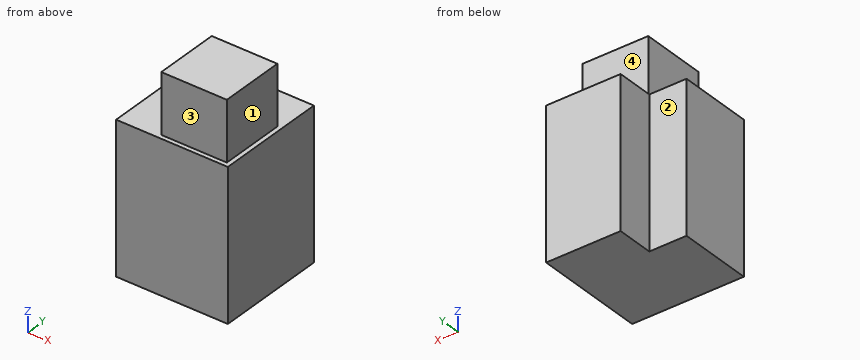
```python
from build123d import *

# Parameters (mm, degrees)
BOX_W              = 10
BOX_H              = 10
BOX_DEPTH          = 10
SKETCH_W           = 4.4
SKETCH_H           = 4.4
PAD_DEPTH          = 4
PAD_FACE4_W        = 10
PAD_FACE4_H        = 10
POCKET_DEPTH       = 2.5
POCKET_FACE5_W     = 10
POCKET_FACE5_H     = 10
POCKET001_DEPTH    = 2.5
SKETCH001_W        = 5
SKETCH001_H        = 10
PAD001_DEPTH       = 10
SKETCH002_W        = 4.4
SKETCH002_H        = 4.4
PAD002_DEPTH       = 4
PAD002_FACE22_W    = 4.4
PAD002_FACE22_H    = 4.4
POCKET002_DEPTH    = 5
POCKET002_FACE16_W = 5
POCKET002_FACE16_H = 10
POCKET003_DEPTH    = 7.5
POCKET003_FACE7_W  = 2.5
POCKET003_FACE7_H  = 10
POCKET004_DEPTH    = 5


with BuildPart() as part:
    # Box → Box (new body)
    with BuildSketch(Plane.XY):
        with Locations((5, 5)):
            Rectangle(BOX_W, BOX_H)
    extrude(amount=BOX_DEPTH)

    # Sketch (on Face6 of BaseFeature) → Pad (new body)
    with BuildSketch(Plane.XY.offset(10)):
        with Locations((5, 5)):
            Rectangle(SKETCH_W, SKETCH_H)
    extrude(amount=PAD_DEPTH)

    # Pad Face4 → Pocket (cut)
    with BuildSketch(Plane(origin=(5, 10, 5), x_dir=(1, 0, 0), z_dir=(0, 1, 0))):
        Rectangle(PAD_FACE4_W, PAD_FACE4_H)
    extrude(amount=-POCKET_DEPTH, mode=Mode.SUBTRACT)

    # Pocket Face5 → Pocket001 (cut)
    with BuildSketch(Plane(origin=(5, 0, 5), x_dir=(-1, 0, 0), z_dir=(0, -1, 0))):
        Rectangle(POCKET_FACE5_W, POCKET_FACE5_H)
    extrude(amount=-POCKET001_DEPTH, mode=Mode.SUBTRACT)

    # Sketch001 (on Face3 of Pocket001) → Pad001 (join)
    with BuildSketch(Plane(origin=(0, 7.5, 0), x_dir=(-1, 0, 0), z_dir=(0, 1, 0))):
        with Locations((-5, 5)):
            Rectangle(SKETCH001_W, SKETCH001_H)
    extrude(amount=PAD001_DEPTH)

    # Sketch002 (on Face6 of Pad001) → Pad002 (join)
    with BuildSketch(Plane.XY.offset(10)):
        with Locations((5, 12.5)):
            Rectangle(SKETCH002_W, SKETCH002_H)
    extrude(amount=PAD002_DEPTH)

    # Pad002 Face22 → Pocket002 (cut)
    with BuildSketch(Plane(origin=(5, 12.5, 14), x_dir=(0, 1, 0), z_dir=(0, 0, 1))):
        Rectangle(PAD002_FACE22_W, PAD002_FACE22_H)
    extrude(amount=-POCKET002_DEPTH, mode=Mode.SUBTRACT)

    # Pocket002 Face16 → Pocket003 (cut)
    with BuildSketch(Plane(origin=(5, 17.5, 5), x_dir=(1, 0, 0), z_dir=(0, 1, 0))):
        Rectangle(POCKET002_FACE16_W, POCKET002_FACE16_H)
    extrude(amount=-POCKET003_DEPTH, mode=Mode.SUBTRACT)

    # Pocket003 Face7 → Pocket004 (cut)
    with BuildSketch(Plane(origin=(8.75, 7.5, 5), x_dir=(1, 0, 0), z_dir=(0, 1, 0))):
        Rectangle(POCKET003_FACE7_W, POCKET003_FACE7_H)
    extrude(amount=-POCKET004_DEPTH, mode=Mode.SUBTRACT)


solid = part.part
```
Work out the finished part from the listing and answer in its coordinate system (mm). Face numbers are marked on the shaded views. A direction names the side the tool comes from. Coordinates: 2 decimals unless noted, no trailing zeros. Loops run counter-clockwise (first coordinate to the right, second up) from the corner with the lowest first, then second, coordinate; pieces in that order, holes last. Notation, with made-up numbers: (35.5, 48.5) -> (58.5, 48.5) arc R17 cw to (58.5, 78.5) -> close; hole circle Ø3 at (59, 8). An arc over 180 degrees is marked (long way). Answer as CSV lines item,"result".
Q1. The part is cut by section A-A on x = 5. Write down the section's boundary in (y, z), and give its area (3 significant figures).
Findings:
outline,"(2.5, 0) -> (10, 0) -> (10, 10) -> (7.2, 10) -> (7.2, 14) -> (2.8, 14) -> (2.8, 10) -> (2.5, 10) -> close"
area,"92.6 mm²"
Q2. The part is cut by section C-C on z = 6.75. Write down the section's boundary in (x, y), and give its area (3 significant figures).
Findings:
outline,"(0, 2.5) -> (7.5, 2.5) -> (7.5, 10) -> (2.5, 10) -> (2.5, 7.5) -> (0, 7.5) -> close"
area,"50.0 mm²"
Q3. A tool of negligible diameter and unlimited length cuts with its end or side. For the marked faces 1, 2, 3 and 4, from which of +Z, -Z, +X, -X, +Y, -Y can it reach the whole face along a straight path? Write none if from no direction.
Findings:
face 1,"+Z, +X, +Y, -Y"
face 2,"+Z, -Z, -X, +Y"
face 3,"+Z, +X, -X, -Y"
face 4,"+Z, +X, -X, +Y"
Q4. Find the intervals of material crossed by probe 1 along Y at (x, z) = (4.75, 11.75); probe 2 along Y at (x, z) = (1.5, 4.5); probe 3 along Z at (x, y) = (3, 7.75), in increasing order.
Findings:
probe 1,"y = 2.8 to 7.2"
probe 2,"y = 2.5 to 7.5"
probe 3,"z = 0 to 10"
Q5. Each of these flat-tipped pins is pushed along its axis until it touches: pin 1 (3 mm diameter, centred on x = 4.5, y = 5.5, fed in from -Z); pin 2 (1.2 mm diameter, centred on x = 1, z = 6, fed in from +Y); pin 3 (3 mm diameter, centred on y = 4, z = 12, fed in from -X); pin 4 (2 mm diameter, centred on x = 4.5, z = 13, fed in from -Y). Where does it stop, or does it pass through?
Findings:
pin 1,"stops at z = 0"
pin 2,"stops at y = 7.5"
pin 3,"stops at x = 2.8"
pin 4,"stops at y = 2.8"
Q6. The part is cut by section D-D on y = 9.25. Write down the section's boundary in (x, z).
Findings:
outline,"(2.5, 0) -> (7.5, 0) -> (7.5, 10) -> (2.5, 10) -> close"
Q7. The part is cut by section B-B on y = 6.25. Write down the section's boundary in (x, z).
Findings:
outline,"(0, 0) -> (7.5, 0) -> (7.5, 10) -> (7.2, 10) -> (7.2, 14) -> (2.8, 14) -> (2.8, 10) -> (0, 10) -> close"
